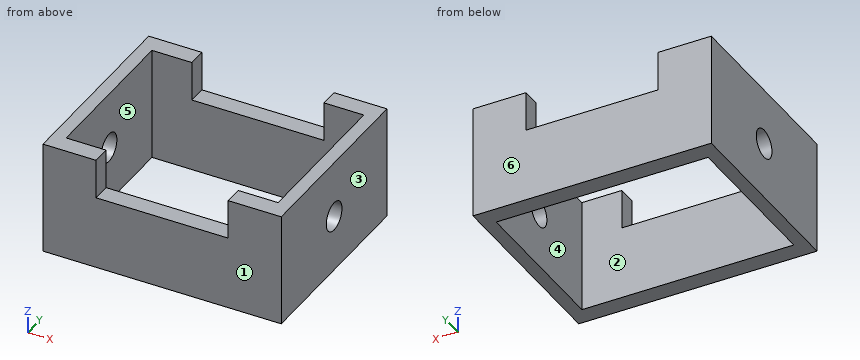
```python
from build123d import *

# Parameters (mm, degrees)
F0_W     = 133.668438
F0_H     = 108.508282
F1_DEPTH = 63.5
F2_R     = 8.039935
F3_DEPTH = 133.669438
F4_W     = 118.878834
F4_H     = 88.022954
F5_DEPTH = 63.501
F6_W     = 74.149776
F6_H     = 22.239236
F7_DEPTH = 108.509281


with BuildPart() as f1:
    # F0 (on Top) → F1 (new body)
    with BuildSketch(Plane.XY):
        Rectangle(F0_W, F0_H)
    extrude(amount=F1_DEPTH)

    # F2 (on face) → F3 (cut, through all)
    with BuildSketch(Plane.YZ.offset(66.834219)):
        with Locations((0, 31.75)):
            Circle(F2_R)
    extrude(amount=-F3_DEPTH, mode=Mode.SUBTRACT)

    # F4 (on face) → F5 (cut, through all)
    with BuildSketch(Plane.XY.offset(63.5)):
        Rectangle(F4_W, F4_H)
    extrude(amount=-F5_DEPTH, mode=Mode.SUBTRACT)

    # F6 (on face) → F7 (cut, through all)
    with BuildSketch(Plane.XZ.offset(54.254141)):
        with Locations((-2e-06, 52.380382)):
            Rectangle(F6_W, F6_H)
    extrude(amount=-F7_DEPTH, mode=Mode.SUBTRACT)


solid = f1.part
```
Could you check a few things on this model? Use its own coordinates, in mm. Face numbers are marked on the shaded views. A direction names the side the tool comes from. Give positions to 0.01 mm unless a question says otherwise; leave off trailing zeros. Order: outer loops, then holes, each group sorted by start corner. A loop starts at its lowest first (then second) coordinate and runs counter-clockwise, first axis right, second up.
Q1. I'm going to push a flat-ended pin straight in: P1, Ø8, axis at x = -6, y = 47.5, coming from the +Z side. Where does the tip first touch, or does it pass through?
Q2. Suppose I cut it at C-C, the plane x = -44. Write out the boundary of the cut face in (y, z).
Q3. Suppose I cut it at D-D, the plane z = 10.5. Write out the boundary of the cut face in (x, y), and give its area (3 significant figures).
Q4. For the marked faces 5 and 6, which set-ups out of +Z, -Z, +X, -X, +Y, -Y let a thin tool reach every point of the face, with its end or its side?
Q5. Suppose I cut it at B-B, the plane y = 10. Write out the boundary of the cut face in (x, z).
Q6. If I drill on line 1 along Y through (x, z) = (22.5, 15.5); line 2 along X through (y, z) = (-27, 45); line 3 along Z through (x, y) = (64, 0), over which ranges is the centre line in solid material (lowest first)?
Q7. We'd pull the mould along Y, two halves only. Please class the marked faces 1, 2, 3 and 4: +Y half, -Y half, draft (parallel to the pull), parting line (faces both ways), or undercut.
Q8. Suppose I cut it at A-A, the plane z = 31.75. Write out the boundary of the cut face in (x, y).
Solution:
1. P1: stops at z = 41.26
2. outline: (-54.25, 0) - (-44.01, 0) - (-44.01, 63.5) - (-54.25, 63.5) - close; (44.01, 0) - (54.25, 0) - (54.25, 63.5) - (44.01, 63.5) - close
3. outline: (-66.83, -54.25) - (66.83, -54.25) - (66.83, 54.25) - (-66.83, 54.25) - close; hole (-59.44, -44.01) - (59.44, -44.01) - (59.44, 44.01) - (-59.44, 44.01) - close
3. area: 4,040 mm2
4. face 5: +Z, -Z
4. face 6: +Z, -Z, +X, -X, +Y
5. outline: (-66.83, 0) - (-59.44, 0) - (-59.44, 63.5) - (-66.83, 63.5) - close; (59.44, 0) - (66.83, 0) - (66.83, 63.5) - (59.44, 63.5) - close
6. line 1: y = -54.25 to -44.01, 44.01 to 54.25
6. line 2: x = -66.83 to -59.44, 59.44 to 66.83
6. line 3: z = 0 to 23.71, 39.79 to 63.5
7. face 1: -Y half
7. face 2: undercut
7. face 3: draft
7. face 4: undercut
8. outline: (-66.83, -54.25) - (66.83, -54.25) - (66.83, -8.04) - (59.44, -8.04) - (59.44, -44.01) - (-59.44, -44.01) - (-59.44, -8.04) - (-66.83, -8.04) - close; (-66.83, 8.04) - (-59.44, 8.04) - (-59.44, 44.01) - (59.44, 44.01) - (59.44, 8.04) - (66.83, 8.04) - (66.83, 54.25) - (-66.83, 54.25) - close
